```python
from build123d import *

# Parameters (mm, degrees)
BOX003_W          = 2.5
BOX003_H          = 57
BOX003_DEPTH      = 25
FILLET_R          = 5
BOX002_W          = 50.5
BOX002_H          = 40.5
BOX002_DEPTH      = 10.3
BOX_W             = 60.5
BOX_H             = 50.5
BOX_DEPTH         = 16.3
BOX001_W          = 63
BOX001_H          = 13.8
BOX001_DEPTH      = 19.4
CYLINDER001_R     = 0.6
CYLINDER001_DEPTH = 10
CYLINDER003_R     = 0.6
CYLINDER003_DEPTH = 10
CYLINDER_R        = 2
CYLINDER_DEPTH    = 1.2
CYLINDER002_R     = 2
CYLINDER002_DEPTH = 1.2
BOX004_W          = 2.5
BOX004_H          = 79
BOX004_DEPTH      = 10.2
FILLET001_R       = 5


with BuildPart() as fillet_body:
    # Box003 → Box003 (new body)
    with BuildSketch(Plane(origin=(-2.5, -3.25, -5.9), x_dir=(1, 0, 0), z_dir=(0, 0, 1))):
        with Locations((1.25, 28.5)):
            Rectangle(BOX003_W, BOX003_H)
    extrude(amount=BOX003_DEPTH)

    # Fillet
    fillet_edges = [fillet_body.edges().sort_by_distance(p)[0] for p in [
        (-1.25, -3.25, -5.9),
        (-1.25, -3.25, 19.1),
        (-1.25, 53.75, -5.9),
        (-1.25, 53.75, 19.1),
    ]]
    fillet(fillet_edges, radius=FILLET_R)


with BuildPart() as cube002:
    # Box002 → Box002 (new body)
    with BuildSketch(Plane(origin=(5, 5, 6), x_dir=(1, 0, 0), z_dir=(0, 0, 1))):
        with Locations((25.25, 20.25)):
            Rectangle(BOX002_W, BOX002_H)
    extrude(amount=BOX002_DEPTH)


with BuildPart() as cube:
    # Box → Box (new body)
    with BuildSketch(Plane.XY):
        with Locations((30.25, 25.25)):
            Rectangle(BOX_W, BOX_H)
    extrude(amount=BOX_DEPTH)


with BuildPart() as cut:
    # Box001 → Box001 (new body)
    with BuildSketch(Plane(origin=(0, 34.4, -3.1), x_dir=(1, 0, 0), z_dir=(0, 0, 1))):
        with Locations((31.5, 6.9)):
            Rectangle(BOX001_W, BOX001_H)
    extrude(amount=BOX001_DEPTH)

    # Fusion: union Cube
    add(cube.part)

    # Cut: cut Cube002
    add(cube002.part, mode=Mode.SUBTRACT)


with BuildPart() as foro:
    # Cylinder001 → Cylinder001 (new body)
    with BuildSketch(Plane(origin=(-6, -8.2, 5), x_dir=(0, 0, -1), z_dir=(1, 0, 0))):
        Circle(CYLINDER001_R)
    extrude(amount=CYLINDER001_DEPTH)


with BuildPart() as foro001:
    # Cylinder003 → Cylinder003 (new body)
    with BuildSketch(Plane(origin=(-6, 58.7, 5), x_dir=(0, 0, -1), z_dir=(1, 0, 0))):
        Circle(CYLINDER003_R)
    extrude(amount=CYLINDER003_DEPTH)


with BuildPart() as cylinder:
    # Cylinder → Cylinder (new body)
    with BuildSketch(Plane(origin=(0, -8.2, 5), x_dir=(0, 0, -1), z_dir=(1, 0, 0))):
        Circle(CYLINDER_R)
    extrude(amount=CYLINDER_DEPTH)


with BuildPart() as cylinder002:
    # Cylinder002 → Cylinder002 (new body)
    with BuildSketch(Plane(origin=(0, 58.7, 5), x_dir=(0, 0, -1), z_dir=(1, 0, 0))):
        Circle(CYLINDER002_R)
    extrude(amount=CYLINDER002_DEPTH)


with BuildPart() as fusion002:
    # Box004 → Box004 (new body)
    with BuildSketch(Plane(origin=(-2.5, -14.3, 0), x_dir=(1, 0, 0), z_dir=(0, 0, 1))):
        with Locations((1.25, 39.5)):
            Rectangle(BOX004_W, BOX004_H)
    extrude(amount=BOX004_DEPTH)

    # Fillet001
    fillet001_edges = [fusion002.edges().sort_by_distance(p)[0] for p in [
        (-1.25, -14.3, 0),
        (-1.25, -14.3, 10.2),
        (-1.25, 64.7, 0),
        (-1.25, 64.7, 10.2),
    ]]
    fillet(fillet001_edges, radius=FILLET001_R)

    # Fusion001: union Cylinder, Cylinder002
    add(cylinder.part)
    add(cylinder002.part)

    # Cut001: cut foro001
    add(foro001.part, mode=Mode.SUBTRACT)

    # Cut002: cut foro
    add(foro.part, mode=Mode.SUBTRACT)

    # Fusion002: union Fillet body, Cut
    add(fillet_body.part)
    add(cut.part)


solid = fusion002.part
```
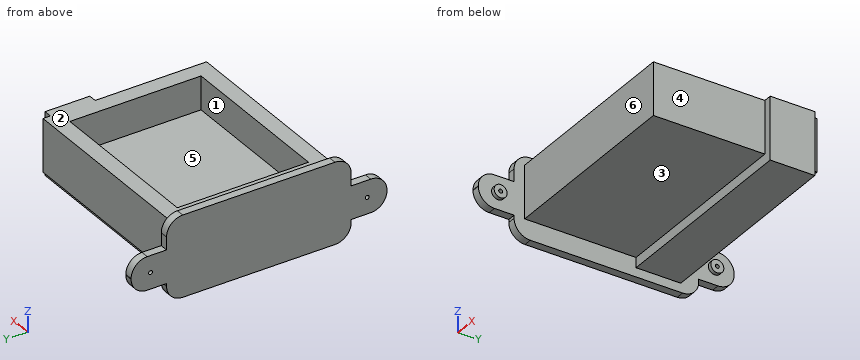
CAD build for the part. Positions are in the model's coordinates, mm. Face numbers are marked on the shaded views. A direction names the side the tool comes from. Round coordinates to 2 decimals unless told otherwise and drop trailing zeros. Loops run counter-clockwise (first coordinate to the right, second up) from the corner with the lowest first, then second, coordinate; pieces in that order, holes last. Notation, with made-up numbers: (13, 1) - (34, 1) arc R8 cw to (34, 5) - close; hole circle Ø8 at (7, 45.5). An arc over 180 degrees is marked (long way). Return JSON: item names as keys, results as strings. Group by question number.
Q1. Drill centre lines: line 1 along Y through (x, z) = (-0.9, 5); line 2 along Y through (x, z) = (10, 10); line 3 along Z through (x, y) = (-0.85, -8.2). Where is each one in solid material? Low to high. Write a range as [from, to].
Q2. Band-saw the part on B-B on x = 58. Give the cut face in (y, z).
Q3. Tool access for the marked faces 1, 2 and 3: list every direction of +Z, -Z, +X, -X, +Y, -Y with a clear straight run to the whole face (end or side of a thin tool).
Q4. Two-plate mould, pull along X, no slides. Class the marked faces 4, 5 and 6: +X half, -X half, draft (parallel to the pull), parting line (faces both ways), or undercut.
Q5. Band-saw the part on C-C on x = 50. Give the cut face in (y, z).
Q6. Band-saw the part on A-A on y = 20. Give the cut face in (x, z), plus the area to 4 significant figures.
Q7. Flat gauge pins, fed straight in: pin 1 Ø3 at (y, z) = (-9, 4) entering from +X; pin 2 Ø13 at (x, z) = (19.5, 4) entering from +Y; pin 3 Ø1.2 at (y, z) = (49, 6.5) entering from +X. Where does each tip first touch, or does it go through?
Solutions:
{
 "1": {"line 1": "y = [-14.3, -8.8], [-7.6, 58.1], [59.3, 64.7]", "line 2": "y = [0, 5], [45.5, 50.5]", "line 3": "z = [0, 4.4], [5.6, 10.2]"},
 "2": {"outline": "(0, 0) - (34.4, 0) - (34.4, -3.1) - (48.2, -3.1) - (48.2, 0) - (50.5, 0) - (50.5, 16.3) - (0, 16.3) - close"},
 "3": {"face 1": "+Z", "face 2": "+Z, +X, +Y, -Y", "face 3": "-Z, +X, -Y"},
 "4": {"face 4": "+X half", "face 5": "undercut", "face 6": "draft"},
 "5": {"outline": "(0, 0) - (34.4, 0) - (34.4, -3.1) - (48.2, -3.1) - (48.2, 0) - (50.5, 0) - (50.5, 16.3) - (45.5, 16.3) - (45.5, 6) - (5, 6) - (5, 16.3) - (0, 16.3) - close"},
 "6": {"outline": "(-2.5, -5.9) - (0, -5.9) - (0, 0) - (60.5, 0) - (60.5, 16.3) - (55.5, 16.3) - (55.5, 6) - (5, 6) - (5, 16.3) - (0, 16.3) - (0, 19.1) - (-2.5, 19.1) - close", "area": "528.5 mm^2"},
 "7": {"pin 1": "stops at x = 1.2", "pin 2": "stops at y = 50.5", "pin 3": "stops at x = 60.5"}
}
